from build123d import *

# Parameters (mm, degrees)
SKETCH_1_R      = 5
SKETCH_1_R_2    = 22
SKETCH_1_R_3    = 17
SKETCH_1_R_4    = 10
EXTRUDE_1_DEPTH = 8
SKETCH_1_3_R    = 17
SKETCH_1_3_R_2  = 10
EXTRUDE_2_DEPTH = 38
SKETCH_2_W      = 13
SKETCH_2_H      = 5


with BuildPart() as part:
    # 草圖1 → 伸長1 (new body)
    # profile 1 of 4: a face of its own
    with BuildSketch(Plane(origin=(0, 0, 0), x_dir=(1, 0, 0), z_dir=(0, 1, 0))):
        with BuildLine():
            Line((33.137931034, 11.263992487), (7.586206897, 20.650652893))
            ThreePointArc((7.586206897, 20.650652893), (18.040185028, 12.591732372), (22, 0))
            ThreePointArc((22, 0), (18.040185028, -12.591732372), (7.586206897, -20.650652893))
            Line((7.586206897, -20.650652893), (33.137931034, -11.263992487))
            ThreePointArc((33.137931034, -11.263992487), (41, 0), (33.137931034, 11.263992487))
        make_face()
        with Locations(Location((29, 0, 0), (0, 0, 270))):
            Circle(SKETCH_1_R, mode=Mode.SUBTRACT)
    # profile 2 of 4: a face of its own
    with BuildSketch(Plane(origin=(0, 0, 0), x_dir=(1, 0, 0), z_dir=(0, 1, 0))):
        Circle(SKETCH_1_R_2)
        Circle(SKETCH_1_R_3, mode=Mode.SUBTRACT)
    # profile 3 of 4: a face of its own
    with BuildSketch(Plane(origin=(0, 0, 0), x_dir=(1, 0, 0), z_dir=(0, 1, 0))):
        Circle(SKETCH_1_R_3)
        with Locations(Location((0, 0, 0), (0, 0, 270))):
            Circle(SKETCH_1_R_4, mode=Mode.SUBTRACT)
    # profile 4 of 4: a face of its own
    with BuildSketch(Plane(origin=(0, 0, 0), x_dir=(1, 0, 0), z_dir=(0, 1, 0))):
        with BuildLine():
            ThreePointArc((-7.586206897, -20.650652893), (-22, 0), (-7.586206897, 20.650652893))
            Line((-7.586206897, 20.650652893), (-33.137931034, 11.263992487))
            ThreePointArc((-33.137931034, 11.263992487), (-41, 0), (-33.137931034, -11.263992487))
            Line((-33.137931034, -11.263992487), (-7.586206897, -20.650652893))
        make_face()
        with Locations(Location((-29, 0, 0), (0, 0, 270))):
            Circle(SKETCH_1_R, mode=Mode.SUBTRACT)
    extrude(amount=EXTRUDE_1_DEPTH)

    # 草圖1<3> → 伸長2 (add)
    with BuildSketch(Plane(origin=(0, 0, 0), x_dir=(1, 0, 0), z_dir=(0, 1, 0))):
        with Locations(Location((0, 0, 0), (0, 0, 270))):
            Circle(SKETCH_1_3_R)
        with Locations(Location((0, 0, 0), (0, 0, 270))):
            Circle(SKETCH_1_3_R_2, mode=Mode.SUBTRACT)
    extrude(amount=EXTRUDE_2_DEPTH)

    # 草圖2 → 除料-旋轉1 (revolve, cut)
    with BuildSketch(Plane.XY, mode=Mode.PRIVATE) as cut_revolve_1_sk:
        with Locations((6.5, 25.5)):
            Rectangle(SKETCH_2_W, SKETCH_2_H)
    revolve(cut_revolve_1_sk.sketch.rotate(Axis((0, 0, 0), (0, 1, 0)), 90), axis=Axis((0, 0, 0), (0, 1, 0)), mode=Mode.SUBTRACT)


solid = part.part
Here's how the part is built. I have some questions about the finished solid (model axes, mm). A direction names the side the tool comes from. Coordinates: 2 decimals unless noted, no trailing zeros. Loops run counter-clockwise (first coordinate to the right, second up) from the corner with the lowest first, then second, coordinate; pieces in that order, holes last.
1. I need wall thicknesses on L1, parallel to Y at x = -4, z = -10.5; L2, parallel to X at y = 25, z = 0; L3, parallel to X at y = 34.25, z = 0. Which ranges of each line are inside material? Lowest first, please.
2. Imagine slicing it at C-C, the plane x = 0. Please give me the cut outline in (y, z).
3. If we mould it in two halves opening along X, with no side actions, what happens to faces 4 (the flat face through (-20.54, 3.94, 15.89)), 5 (the cylindrical face through (-9.76, 32.93, -2.17)), 6 (the cylindrical face through (0, 4, -22)), 7 (the cylindrical face through (7.91, 25.535, 10.316))? For each: pulls with the +X half, pulls with the -X half, needs draft (parallel to the pull), parting line crosses it, or undercut.
4. For faces 1 (the cylindrical face through (41, 4, 0)), 2 (the flat face through (8, 28, 7)), 3 (the cylindrical face through (16.855, 22.79, -2.213)), which set-ups out of +Z, -Z, +X, -X, +Y, -Y let a thin tool reach every point of the face, with its end or its side?
5. Imagine slicing it at B-B, the plane z = 0. Please give me the cut outline in (x, y).
6. For P1, Ø6, axis at x = -30.5, y = 6, coming from the -Z side; P2, Ø4, axis at y = 28.5, z = 0.5, coming from the -X side; P3, Ø11.5, axis at x = -29, z = 0, coming from the +Y side; P4, Ø13, axis at x = -4, z = 5.5, coming from the -Y side, each with a flat end and sliding along its axis, tell me the tip position at first contact or that it passes through.
7. Imagine slicing it at A-A, the plane y = 6. Please give me the cut outline in (x, z).
8. Imagine slicing it at D-D, the plane z = 6.5. Please give me the cut outline in (x, y).
Taken from the geometry:
1. L1: y = 0 to 23, 28 to 38
1. L2: x = -17 to -13, 13 to 17
1. L3: x = -17 to -10, 10 to 17
2. outline: (0, -22) - (8, -22) - (8, -17) - (38, -17) - (38, -10) - (28, -10) - (28, -13) - (23, -13) - (23, -10) - (0, -10) - close; (0, 10) - (23, 10) - (23, 13) - (28, 13) - (28, 10) - (38, 10) - (38, 17) - (8, 17) - (8, 22) - (0, 22) - close
3. face 4: pulls with the -X half
3. face 5: undercut
3. face 6: parting line crosses it
3. face 7: undercut
4. face 1: +X, +Y, -Y
4. face 2: none
4. face 3: +Y
5. outline: (-41, 0) - (-34, 0) - (-34, 8) - (-41, 8) - close; (-24, 0) - (-10, 0) - (-10, 23) - (-13, 23) - (-13, 28) - (-10, 28) - (-10, 38) - (-17, 38) - (-17, 8) - (-24, 8) - close; (10, 0) - (24, 0) - (24, 8) - (17, 8) - (17, 38) - (10, 38) - (10, 28) - (13, 28) - (13, 23) - (10, 23) - close; (34, 0) - (41, 0) - (41, 8) - (34, 8) - close
6. P1: stops at z = -13.34
6. P2: stops at x = -17
6. P3: stops at y = 8
6. P4: stops at y = 0
7. outline: (-33.14, -11.26) - (-7.59, -20.65) arc R22 ccw to (7.59, -20.65) - (33.14, -11.26) arc R12 ccw to (33.14, 11.26) - (7.59, 20.65) arc R22 ccw to (-7.59, 20.65) - (-33.14, 11.26) arc R12 ccw to start; hole circle Ø10 at (-29, 0); hole circle Ø20 at (0, 0); hole circle Ø10 at (29, 0)
8. outline: (-39.09, 0) - (-7.6, 0) - (-7.6, 23) - (-11.26, 23) - (-11.26, 28) - (-7.6, 28) - (-7.6, 38) - (-15.71, 38) - (-15.71, 8) - (-39.09, 8) - close; (7.6, 0) - (39.09, 0) - (39.09, 8) - (15.71, 8) - (15.71, 38) - (7.6, 38) - (7.6, 28) - (11.26, 28) - (11.26, 23) - (7.6, 23) - close
